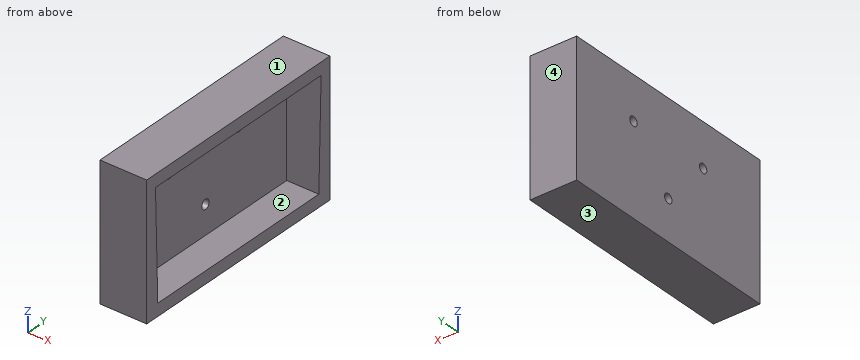
from build123d import *

# Parameters (mm, degrees)
SKETCH1_W           = 129
SKETCH1_H           = 74
BOSS_EXTRUDE1_DEPTH = 39
SKETCH3_R           = 1.5
CUT_EXTRUDE2_DEPTH  = 10
CAVITY1_START       = 3.561625
CAVITY1_DEPTH       = 66.86575
CAVITY1_START_2     = 3
CAVITY1_2_DEPTH     = 123
SKETCH4_W           = 114
SKETCH4_H           = 39
CUT_EXTRUDE3_DEPTH  = 100
SKETCH5_W           = 15
SKETCH5_H           = 74
BOSS_EXTRUDE2_DEPTH = 4


with BuildPart() as part:
    # Sketch1 → Boss-Extrude1 (new body)
    with BuildSketch(Plane.XY):
        with Locations((64.5, 37)):
            Rectangle(SKETCH1_W, SKETCH1_H)
    extrude(amount=-BOSS_EXTRUDE1_DEPTH)

    # Sketch3 → Cut-Extrude2 (cut)
    with BuildSketch(Plane.ZY):
        with Locations((-10, 51.05)):
            Circle(SKETCH3_R)
        with Locations((-10, 22.95)):
            Circle(SKETCH3_R)
        with Locations((-26, 37)):
            Circle(SKETCH3_R)
    extrude(amount=-CUT_EXTRUDE2_DEPTH, mode=Mode.SUBTRACT)

    # Cavity1: read off the stored shape, not the designer's step
    # Cavity1 outline → Cavity1 (cut)
    with BuildSketch(Plane(origin=(0, 0, 0), x_dir=(1, 0, 0), z_dir=(0, 1, 0)).offset(CAVITY1_START)):
        Polygon((124.330201477, 35.035), (4.664798523, 35.035), (3.746, 0), (125.249, 0), align=None)
    extrude(amount=CAVITY1_DEPTH, mode=Mode.SUBTRACT)

    # Cavity1 2 outline → Cavity1 2 (add)
    with BuildSketch(Plane.YZ.offset(CAVITY1_START_2)):
        Polygon((70.427375, 0), (69.505826955, -35.035), (70.427375, -35.035), align=None)
        Polygon((4.483173045, -35.035), (3.561625, 0), (3.561625, -35.035), align=None)
    extrude(amount=CAVITY1_2_DEPTH)

    # Sketch4 → Cut-Extrude3 (cut)
    with BuildSketch(Plane(origin=(0, 74, 0), x_dir=(1, 0, 0), z_dir=(0, 1, 0))):
        with Locations((72, 19.5)):
            Rectangle(SKETCH4_W, SKETCH4_H)
    extrude(amount=-CUT_EXTRUDE3_DEPTH, mode=Mode.SUBTRACT)

    # Sketch5 → Boss-Extrude2 (add)
    with BuildSketch(Plane.XY):
        with Locations((7.5, 37)):
            Rectangle(SKETCH5_W, SKETCH5_H)
    extrude(amount=BOSS_EXTRUDE2_DEPTH)


solid = part.part
Model file for the job. Use its own axes, mm. Face numbers are marked on the shaded views. Coordinates: 2 decimals unless noted, no trailing zeros. Order: outer loops, then holes, each group sorted by start corner. A loop starts at its lowest first (then second) coordinate and runs counter-clockwise, first axis right, second up. Notation, with made-up numbers: (28, -16.5) -> (42, -16.5) arc R26 ccw to (42, -0.5) -> close; hole circle Ø7 at (46, 80.5). An arc over 180 degrees is marked (long way). Return JSON: item names as keys, results as strings. Group by question number.
Item 1: Saw through at B-B on y = 10. Write the cut outline in (x, z) (3 decimals).
Item 2: Saw through at A-A on x = 9.75. Write the cut outline in (y, z) (3 decimals).
Item 3: Flat gauge pins, fed straight in: P1, Ø8, axis at y = 28, z = -19, coming from the +X side; P2, Ø3, axis at x = 13, z = -17, coming from the -Y side; P3, Ø4, axis at y = 49, z = -13.5, coming from the +X side; P4, Ø5, axis at y = 22.95, z = -10, coming from the +X side. Where does each tip first touch, or does it go through?
Item 4: Saw through at D-D on z = -10. Write the cut outline in (x, y).
Item 5: Pull direction Z, two halves, no side cores. Call the marked faces 1, 2, 3 and 4: pulls with the +Z half, pulls with the -Z half, needs draft (parallel to the pull), parting line crosses it, or undercut.
Item 6: Wall check: line 1 along Y through (x, z) = (2.65, -10); line 2 along Z through (x, y) = (9.25, 54) (3 decimals); line 3 along Y through (x, z) = (1.7, -26). Give the ranges that are in metal, low to high. Write a range as [from, to].
Item 7: Saw through at C-C on y = 51.05. Write the cut outline in (x, z) (3 decimals).
Values found:
{
 "1": {"outline": "(0, -39) -> (15, -39) -> (15, -35.035) -> (4.665, -35.035) -> (3.746, 0) -> (15, 0) -> (15, 4) -> (0, 4) -> close"},
 "2": {"outline": "(0, -39) -> (74, -39) -> (74, 4) -> (0, 4) -> close; hole (3.562, 0) -> (4.483, -35.035) -> (69.506, -35.035) -> (70.427, 0) -> close"},
 "3": {"P1": "stops at x = 4.35", "P2": "stops at y = 0", "P3": "stops at x = 4.15", "P4": "stops at x = 4.07"},
 "4": {"outline": "(0, 0) -> (15, 0) -> (15, 3.82) -> (4.01, 3.82) -> (4.01, 21.45) -> (0, 21.45) -> close; (0, 24.45) -> (4.01, 24.45) -> (4.01, 49.55) -> (0, 49.55) -> close; (0, 52.55) -> (4.01, 52.55) -> (4.01, 70.16) -> (15, 70.16) -> (15, 74) -> (0, 74) -> close"},
 "5": {"face 1": "pulls with the +Z half", "face 2": "undercut", "face 3": "pulls with the -Z half", "face 4": "needs draft"},
 "6": {"line 1": "y = [0, 21.45], [24.45, 49.55], [52.55, 74]", "line 2": "z = [-39, -35.035], [0, 4]", "line 3": "y = [0, 35.5], [38.5, 74]"},
 "7": {"outline": "(0, -39) -> (15, -39) -> (15, -35.035) -> (4.665, -35.035) -> (4.048, -11.5) -> (0, -11.5) -> close; (0, -8.5) -> (3.969, -8.5) -> (3.746, 0) -> (15, 0) -> (15, 4) -> (0, 4) -> close"}
}
